Autodesk Inventor part; units mm, degrees
ref_plane "YZ Plane" through (0, 0, 0) normal (1, 0, 0) x (0, 1, 0)
ref_plane "XZ Plane" through (0, 0, 0) normal (0, 1, 0) x (-1, 0, 0)
ref_plane "XY Plane" through (0, 0, 0) normal (0, 0, 1) x (1, 0, 0)
sketch "Sketch1" plane through (0, 0, 0) normal (1, 0, 0) x (0, 1, 0)
  line L0 (-66.294, 254) -> (66.294, 254)
  line L1 (66.294, 254) -> (66.294, -254)
  line L2 (66.294, -254) -> (-66.294, -254)
  line L3 (-66.294, -254) -> (-66.294, 254)
  line L4 (-66.294, 254) -> (66.294, -254) construction
  line L5 (66.294, 254) -> (-66.294, -254) construction
  point P0 (0, 0)
  dimension "d0" = 508
  dimension "d1" = 132.588
extrude "Extrusion1" add sketch "Sketch1" along normal blind 3.175
sketch "Sketch2" plane through (3.175, 0, 0) normal (1, 0, 0) x (0, 0, -1)
  line L0 (-67.5894, -66.294) -> (67.691, -66.294) construction
  line L1 (67.691, -66.294) -> (67.691, -22.098) construction
  line L2 (67.691, -22.098) -> (-67.5894, -22.098) construction
  line L3 (-67.5894, -22.098) -> (-67.5894, -66.294) construction
  line L4 (-67.5894, -66.294) -> (67.691, -22.098) construction
  line L5 (67.691, -66.294) -> (-67.5894, -22.098) construction
  line L6 (254, -66.294) -> (254, 66.294) construction
  line L7 (-254, -66.294) -> (254, -66.294) construction
  point P0 (0, 0)
  point P1 (0.0508, -44.196)
  point P2 (10.6003, -66.294)
  dimension "d4" = 135.2804
  dimension "d5" = 44.196
  dimension "d6" = 186.309
sketch "Sketch3" plane through (3.175, 0, 0) normal (1, 0, 0) x (0, 0, -1)
  line L0 (-33.7566, -40.005) -> (33.8582, -40.005) construction
  line L1 (-254, -66.294) -> (254, -66.294) construction
  line L2 (67.691, -66.294) -> (67.691, -22.098) construction
  line L3 (-67.5894, -22.098) -> (-67.5894, -66.294) construction
  point P0 (0, 0)
  dimension "d7" = 26.289
  dimension "d17" = 33.8328
  dimension "d18" = 33.8328
hole "Hole1" at (3.175, -40.005, 33.7566) at (3.175, -40.005, -33.8582) direction (-1, 0, 0) diameter 4.4958 end through all
sketch "brackets" plane through (3.175, 0, 0) normal (1, 0, 0) x (0, 0, -1)
  line L0 (254, -66.294) -> (254, 66.294) construction
  line L1 (249.428, 54.61) -> (230.378, 54.61) construction
  line L2 (230.378, 54.61) -> (230.378, -54.61) construction
  line L3 (230.378, -54.61) -> (249.428, -54.61) construction
  line L4 (249.428, -54.61) -> (249.428, 54.61) construction
  line L5 (254, 66.294) -> (-254, 66.294) construction
  line L6 (-254, 66.294) -> (-254, -66.294) construction
  line L7 (-249.428, 54.61) -> (-230.378, 54.61) construction
  line L8 (-230.378, 54.61) -> (-230.378, -54.61) construction
  line L9 (-230.378, -54.61) -> (-249.428, -54.61) construction
  line L10 (-249.428, -54.61) -> (-249.428, 54.61) construction
  point P0 (0, 0)
  point P1 (-236.3724, 29.21)
  point P2 (-236.3724, -29.21)
  point P3 (236.3724, 29.21)
  point P4 (236.3724, -29.21)
  dimension "d20" = 19.05
  dimension "d21" = 109.22
  dimension "d22" = 11.684
  dimension "d23" = 19.05
  dimension "d24" = 109.22
  dimension "d25" = 11.684
  dimension "d26" = 25.4
  dimension "d27" = 5.9944
  dimension "d28" = 25.4
  dimension "d29" = 5.9944
  dimension "d30" = 25.4
  dimension "d31" = 5.9944
  dimension "d32" = 25.4
  dimension "d33" = 5.9944
  dimension "d41" = 4.572
  dimension "d42" = 4.572
hole "Hole2" at (3.175, 29.21, 236.3724) at (3.175, -29.21, 236.3724) at (3.175, 29.21, -236.3724) at (3.175, -29.21, -236.3724) direction (-1, 0, 0) diameter 4.2926 end through all countersink diameter 9.398 countersink angle 90
properties part number "nmt_sidepanel_20in"
Input: part model. Units: mm. Frame: model coordinates. Coordinates: 2 decimals unless noted, no trailing zeros. Answer as a JSON object with one key per item and string values.
1. First-contact query: P1, Ø4, axis at y = -40.01, z = -33.86, coming from the +X side. Flat tip, straight axial feed; report the tip coordinate or a pass-through.
Result set:
{"P1": "passes through"}
2. Mould query, pull axis Y, two halves, no side actions, for faces 1 (the face through (0, -1, 4)), 2 (the face through (0.782, -28.517, 234.173)). Classes: released by +Y, released by -Y, zero draft, split by the parting line, or undercut.
Result set:
{"face 1": "zero draft", "face 2": "undercut"}
3. Material intervals for line 1 (Z direction, x = 0.3, y = -29.21); line 2 (Z direction, x = 2.05, y = 29), sorted ascending. Write a range as from..to.
Result set:
{"line 1": "z = -254..-238.52, -234.23..234.23, 238.52..254", "line 2": "z = -254..-239.94, -232.8..232.8, 239.94..254"}
